Here's the drawing with two shaded views (mm, measured from the low corner). I have some questions. A direction names the side the tool comes from. Coordinates: 2 decimals unless noted, no trailing zeros. Write each loop counter-clockwise with the first axis right and the second up, starting at its lowest first coordinate (ties: lowest second). Pieces come first, ordered by that corner, then holes. Notation, with made-up numbers: M 66,-32 L 80,-32 A34 ccw 80,2 Z; hole C 75,30 d5. An arc over 180 degrees is marked long. Answer as CSV lines item,"result". Start each with the question number.
Item 1: Suppose I cut it at C-C, the plane y = 4.75. Write out the boundary of the cut face in (x, z).
Item 2: Suppose I cut it at B-B, the plane x = 12.25. Write out the boundary of the cut face in (y, z), and give its area (3 significant figures).
Item 3: Suppose I cut it at A-A, the plane z = 1. Write out the boundary of the cut face in (x, y).
Item 4: I'm going to push a flat-ended pin straight in: P1, Ø0.6, axis at y = 11, z = 1, coming from the -X side. Where does the tip first touch, or does it pass through?
Item 5: On a 3-axis mill with a long thin cutter (end or side, diameter ignored), from which of +Z, -Z, +X, -X, +Y, -Y can I reach the whole of each face in a straight line? I mean the marked faces 1, 2 and 3. Say none if no direction works.
Item 6: If I drill on line 1 along X through (y, z) = (3, 0.65); line 2 along Y through (x, z) = (12, 0.8); line 3 along X through (y, z) = (16.25, 1.05), over which ranges is the centre line in solid material (lowest first)? Write a range as [from, to].
Item 7: Suppose I cut it at D-D, the plane x = 1.75. Write out the boundary of the cut face in (y, z).
Item 8: We'd pull the mould along Y, two halves only. Please class the marked faces 4, 5, 6 and 7: +Y half, -Y half, draft (parallel to the pull), parting line (faces both ways), or undercut.
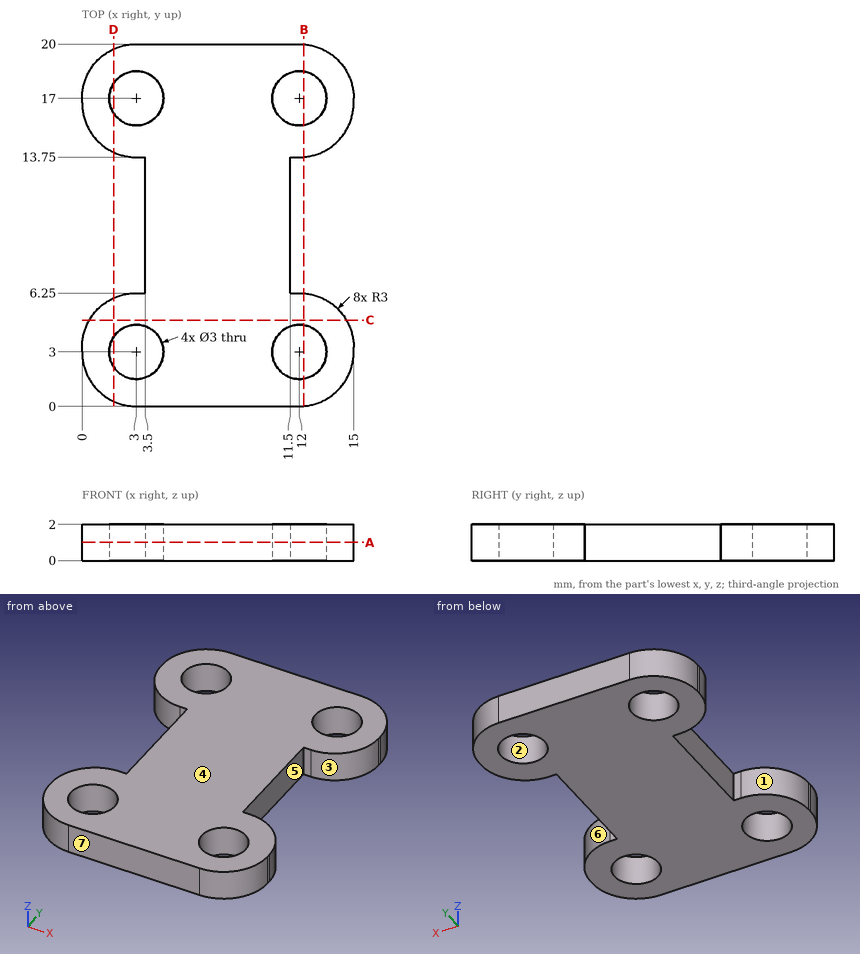
Ans:
1,outline,"M 0.4,0 L 14.6,0 L 14.6,2 L 0.4,2 Z"
2,outline,"M 0.01,0 L 1.52,0 L 1.52,2 L 0.01,2 Z; M 4.48,0 L 6.24,0 L 6.24,2 L 4.48,2 Z; M 13.76,0 L 15.52,0 L 15.52,2 L 13.76,2 Z; M 18.48,0 L 19.99,0 L 19.99,2 L 18.48,2 Z"
2,area,"13.1 mm^2"
3,outline,"M 0,3 A3 ccw 3,0 L 12,0 A3 ccw 15,3 L 15,3.25 A3 ccw 12,6.25 L 11.5,6.25 L 11.5,13.75 L 12,13.75 A3 ccw 15,16.75 L 15,17 A3 ccw 12,20 L 3,20 A3 ccw 0,17 L 0,16.75 A3 ccw 3,13.75 L 3.5,13.75 L 3.5,6.25 L 3,6.25 A3 ccw 0,3.25 Z; hole C 3,3 d3; hole C 3,17 d3; hole C 12,3 d3; hole C 12,17 d3"
4,P1,"stops at x = 3.5"
5,face 1,"+Z, -Z, -X"
5,face 2,"+Z, -Z"
5,face 3,"+Z, -Z, +X"
6,line 1,"x = [0, 1.5], [4.5, 10.5], [13.5, 15]"
6,line 2,"y = [0, 1.5], [4.5, 6.25], [13.75, 15.5], [18.5, 20]"
6,line 3,"x = [0.04, 1.7], [4.3, 10.7], [13.3, 14.96]"
7,outline,"M 0.27,0 L 2.17,0 L 2.17,2 L 0.27,2 Z; M 3.83,0 L 5.98,0 L 5.98,2 L 3.83,2 Z; M 14.02,0 L 16.17,0 L 16.17,2 L 14.02,2 Z; M 17.83,0 L 19.73,0 L 19.73,2 L 17.83,2 Z"
8,face 4,"draft"
8,face 5,"undercut"
8,face 6,"undercut"
8,face 7,"-Y half"
